```python
from build123d import *

# Parameters (mm, degrees)
F1_DEPTH = 1.2
F3_DEPTH = 12.5
F5_DEPTH = 2


with BuildPart() as f1:
    # F0 (on Top) → F1 (new body)
    with BuildSketch(Plane.XY):
        with BuildLine():
            ThreePointArc((-3.25, -2.331845), (0, 4), (3.25, -2.331845))
            Line((3.25, -2.331845), (4.177124, -3.831845))
            Line((4.177124, -3.831845), (5.5, -2.331845))
            Line((5.5, -2.331845), (6.286185, 8.410343))
            ThreePointArc((6.286185, 8.410343), (0, 10.5), (-6.286185, 8.410343))
            Line((-6.286185, 8.410343), (-5.5, -2.331845))
            Line((-5.5, -2.331845), (-4.177124, -3.831845))
            Line((-4.177124, -3.831845), (-3.25, -2.331845))
        make_face()
    extrude(amount=F1_DEPTH)

    # F2 (on Right) → F3 (cut, symmetric)
    with BuildSketch(Plane.YZ):
        Polygon((-3.831845, 0.4), (-2.331845, 1.2), (-3.831845, 1.2), align=None)
    extrude(amount=F3_DEPTH, both=True, mode=Mode.SUBTRACT)

    # F4 (on face) → F5 (join)
    with BuildSketch(Plane.XY.offset(1.2)):
        with BuildLine():
            ThreePointArc((5.167966, 6.106728), (2.751924, 7.511785), (0, 8))
            ThreePointArc((0, 8), (-2.751924, 7.511785), (-5.167966, 6.106728))
            ThreePointArc((-5.167966, 6.106728), (-5.238273, 5.968098), (-5.188072, 5.820989))
            Line((-5.188072, 5.820989), (-4.324815, 4.852419))
            Line((-4.324815, 4.852419), (-4.238297, 4.755347))
            ThreePointArc((-4.238297, 4.755347), (-4.116589, 4.690331), (-3.981744, 4.719604))
            Line((-3.981744, 4.719604), (-2.605887, 5.593689))
            ThreePointArc((-2.605887, 5.593689), (-2.51793, 5.718968), (-2.544321, 5.86975))
            Line((-2.544321, 5.86975), (-2.599979, 5.957358))
            ThreePointArc((-2.599979, 5.957358), (-1.328001, 6.362893), (0, 6.5))
            ThreePointArc((0, 6.5), (1.328001, 6.362893), (2.599979, 5.957358))
            Line((2.599979, 5.957358), (2.544321, 5.86975))
            ThreePointArc((2.544321, 5.86975), (2.51793, 5.718968), (2.605887, 5.593689))
            Line((2.605887, 5.593689), (3.981744, 4.719604))
            ThreePointArc((3.981744, 4.719604), (4.116589, 4.690331), (4.238297, 4.755347))
            Line((4.238297, 4.755347), (4.324815, 4.852419))
            Line((4.324815, 4.852419), (5.188072, 5.820989))
            ThreePointArc((5.188072, 5.820989), (5.238273, 5.968098), (5.167966, 6.106728))
        make_face()
    extrude(amount=F5_DEPTH)


solid = f1.part
```
Work out the finished part from the listing and answer in its coordinate system (mm). A direction names the side the tool comes from. Coordinates: 2 decimals unless noted, no trailing zeros. Write each loop counter-clockwise with the first axis right and the second up, starting at its lowest first coordinate (ties: lowest second). Pieces come first, ordered by that corner, then holes.
Q1. A cutting plane is placed at A-A, the plane y = 0. Give the vertices of the cut face in (x, z), then the cut area to 3 significant figures.
Q2. Find the intervals of material crossed by line 1 (X direction, y = 0, z = 0.75); line 2 (Z direction, x = -0.5, y = 9.75); line 3 (Y direction, x = 0, z = 0.95), in increasing order.
Q3. Which of the six approach directions +Z, -Z, +X, -X, +Y, -Y give full straight-line access (tool end or side, diameter ignored) to faces 1 (the face through (-3.303, 5.151, 2.186)), 2 (the face through (0, 6, 1.2)), 3 (the face through (3.6, -2.9, 0.5))?
Q4. A cutting plane is placed at D-D, the plane y = 5.25. Give the vertices of the cut face in (x, z), then the cut area to 3 significant figures.
Q5. Determine the mould class of faces 4 (the face through (-3.6, -2.9, 0.5)), 5 (the face through (4.39, -2.76, 0.97)), 6 (the face through (5.888, 2.964, 0.592)) for opening direction X: released by +X, released by -X, zero draft, split by the parting line, or undercut.
Q6. A cutting plane is placed at B-B, the plane z = 2.7. Give the vertices of the cut face in (x, y).
Q7. This flat-tipped pin is pushed along its axis until it touches: pin 1 Ø1 at (x, z) = (3.5, 1.5) entering from -Y. Where does it stop, or does it pass through?
Q8. A cutting plane is placed at C-C, the plane x = 2. Give the vertices of the cut face in (y, z), then the cut area to 3 significant figures.
Findings below:
1. outline: (-5.67, 0) - (-4, 0) - (-4, 1.2) - (-5.67, 1.2) - close; (4, 0) - (5.67, 0) - (5.67, 1.2) - (4, 1.2) - close
1. area: 4.01 mm2
2. line 1: x = -5.67 to -4, 4 to 5.67
2. line 2: z = 0 to 1.2
2. line 3: y = 4 to 10.5
3. face 1: +Z, -Y
3. face 2: +Z
3. face 3: +Z, -Z, -Y
4. outline: (-6.05, 0) - (6.05, 0) - (6.05, 1.2) - (4.68, 1.2) - (4.68, 3.2) - (3.15, 3.2) - (3.15, 1.2) - (-3.15, 1.2) - (-3.15, 3.2) - (-4.68, 3.2) - (-4.68, 1.2) - (-6.05, 1.2) - close
4. area: 20.7 mm2
5. face 4: undercut
5. face 5: zero draft
5. face 6: released by +X
6. outline: (-5.19, 5.82) - (-4.32, 4.85) - (-4.24, 4.76) arc R0.2 ccw to (-3.98, 4.72) - (-2.61, 5.59) arc R0.2 ccw to (-2.54, 5.87) - (-2.6, 5.96) arc R6.5 cw to (0, 6.5) arc R6.5 cw to (2.6, 5.96) - (2.54, 5.87) arc R0.2 ccw to (2.61, 5.59) - (3.98, 4.72) arc R0.2 ccw to (4.24, 4.76) - (4.32, 4.85) - (5.19, 5.82) arc R0.2 ccw to (5.17, 6.11) arc R8 ccw to (-5.17, 6.11) arc R0.2 ccw to start
7. pin 1: stops at y = -2.71
8. outline: (3.46, 0) - (10.31, 0) - (10.31, 1.2) - (7.75, 1.2) - (7.75, 3.2) - (6.18, 3.2) - (6.18, 1.2) - (3.46, 1.2) - close
8. area: 11.3 mm2
